```python
from build123d import *

# Parameters (mm, degrees)
SKETCH_2_R          = 6.5
CUT_EXTRUDE_1_DEPTH = 38.749172176


with BuildPart() as part:
    # Эскиз1 → Повернуть1 (revolve)
    with BuildSketch(Plane(origin=(0, 0, 0), x_dir=(0, 0, -1), z_dir=(1, 0, 0)), mode=Mode.PRIVATE) as revolve_1_sk:
        with BuildLine():
            Line((0, 8), (0, 10))
            Line((0, 10), (-13.5, 10))
            ThreePointArc((-13.5, 10), (-14.58559515, 8.794493938), (-16, 8))
            Line((-16, 8), (-16, 0))
            Line((-16, 0), (19, 0))
            Line((19, 0), (19, 8))
            Line((19, 8), (0, 8))
        make_face()
    revolve(revolve_1_sk.sketch.rotate(Axis((0, 0, 16), (0, 0, -1)), 90), axis=Axis((0, 0, 16), (0, 0, -1)))

    # Эскиз2 → Вырез-Вытянуть1 (cut, through all)
    with BuildSketch(Plane.XY.offset(16)):
        Circle(SKETCH_2_R)
    extrude(amount=-CUT_EXTRUDE_1_DEPTH, mode=Mode.SUBTRACT)


solid = part.part
```
Source: CAD feature listing. Evaluate the final solid. Frame: model axes, mm. A direction names the side the tool comes from. Give positions to 0.01 mm unless a question says otherwise; leave off trailing zeros. Loops run counter-clockwise (first coordinate to the right, second up) from the corner with the lowest first, then second, coordinate; pieces in that order, holes last. Notation, with made-up numbers: M 29,8 L 53,8 A16 ccw 53,12 Z; hole C 16.5,-33.75 d10. An arc over 180 degrees is marked long. Put each result on its own line as item: value.
Q1. Section D-D (z = 1). Return the cut outline in (x, y).
Response values:
outline: C 0,0 d20; hole C 0,0 d13
Q2. Section C-C (z = -5). Return the cut outline in (x, y).
Response values:
outline: C 0,0 d16; hole C 0,0 d13
Q3. Mould query, pull axis X, two halves, no side actions, for faces 3 (the cylindrical face through (-5.158, -3.955, -1.255)), 4 (the flat face through (0, -7, -19)), 5 (the cylindrical face through (-10, 0, 7)). Classes: released by +X, released by -X, zero draft, split by the parting line, or undercut.
Response values:
face 3: undercut
face 4: zero draft
face 5: split by the parting line
Q4. Line query: probe 1 along Y at (x, z) = (0, 6); probe 2 along Y at (x, z) = (0, -7); probe 3 along X at (y, z) = (-2.75, -15.5). Output: solid intervals per line, ascending. Write a range as [from, to].
Response values:
probe 1: y = [-10, -6.5], [6.5, 10]
probe 2: y = [-8, -6.5], [6.5, 8]
probe 3: x = [-7.51, -5.89], [5.89, 7.51]
Q5. Section A-A (x = 0). Return the cut outline in (y, z), and give its area (3 significant figures).
Response values:
outline: M -10,0 L -8,0 L -8,-19 L -6.5,-19 L -6.5,16 L -8,16 A5 cw -10,13.5 Z; M 6.5,-19 L 8,-19 L 8,0 L 10,0 L 10,13.5 A5 cw 8,16 L 6.5,16 Z
area: 163 mm²
Q6. Pin query (flat end, axial travel): P1, Ø8, axis at x = -2.5, z = -15, coming from the +Y side; P2, Ø1.5, axis at y = 7.5, z = 7.5, coming from the -X side; P3, Ø4, axis at y = 3.5, z = -12, coming from the +X side. Return the tip coordinate at first contact, or that it passes through.
Response values:
P1: stops at y = 8
P2: stops at x = -7.38
P3: stops at x = 7.86
Q7. Reachability of faces 1 (the flat face through (0, -7, 16)), 2 (the flat face through (0, -8.2, 0)) from +Z, -Z, +X, -X, +Y, -Y: full face, straight path, thin tool, end or side. Return the list, or none.
Response values:
face 1: +Z, +X, -X, +Y, -Y
face 2: -Z
